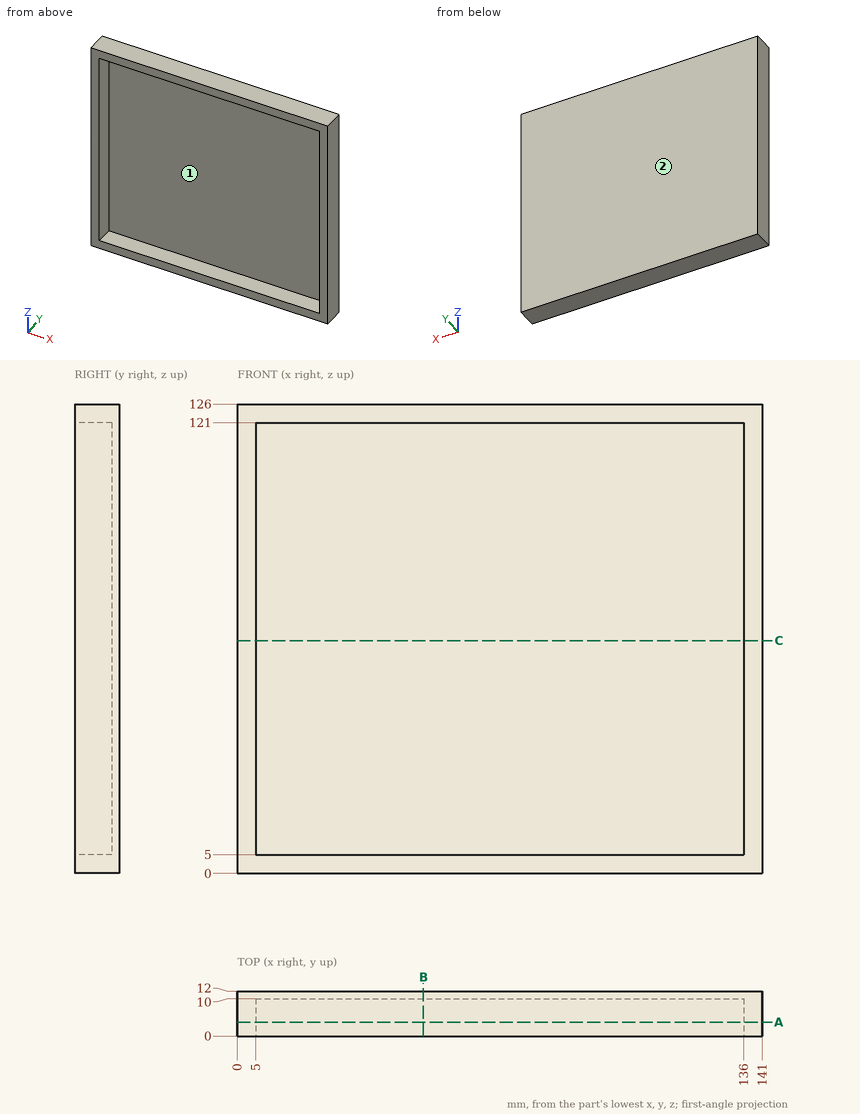
Input: dimensioned drawing with shaded views. Units: mm. Origin: part minimum x, y, z. Give positions to 0.01 mm unless a question says otherwise; leave off trailing zeros. Loops run counter-clockwise (first coordinate to the right, second up) from the corner with the lowest first, then second, coordinate; pieces in that order, holes last. Notation, with made-up numbers: M 18,46.5 L 56,46.5 A17 ccw 56,72.5 Z; hole C 74.25,-35.75 d10. An arc over 180 degrees is marked long. Put each result on its own line as item: value. Start each with the question number.
1) Cut plane A-A (y = 3.75). Output: boundary loops of the cut face in (x, z), then the cut area to 3 significant figures.
2) Ray query, line 1 along X through (y, z) = (6, 44); line 2 along Z through (x, y) = (105, 2.5); line 3 along Y through (x, z) = (110, 100). Return the intervals inside material, ascending.
3) Contact query for flat-ended pins moving along their axis: pin 1 (1.5 mm diameter, centred on y = 4, z = 55.5, fed in from -X); pin 2 (5 mm diameter, centred on x = 62.5, z = 95.5, fed in from -Y). Output: stop coordinate, or through.
4) Cut plane B-B (x = 50). Output: boundary loops of the cut face in (y, z).
5) Cut plane C-C (z = 62.5). Output: boundary loops of the cut face in (x, y), then the cut area to 3 significant figures.
6) Pull-direction query (Z, two-part tool) for the marked faces 1 and 2; classes: pulls with the +Z half, pulls with the -Z half, needs draft (parallel to the pull), parting line crosses it, or undercut.
Verdict:
1. outline: M 0,0 L 141,0 L 141,126 L 0,126 Z; hole M 5,5 L 136,5 L 136,121 L 5,121 Z
1. area: 2,570 mm2
2. line 1: 0 to 5, 136 to 141
2. line 2: 0 to 5, 121 to 126
2. line 3: 10 to 12
3. pin 1: x = 0
3. pin 2: y = 10
4. outline: M 0,0 L 12,0 L 12,126 L 0,126 L 0,121 L 10,121 L 10,5 L 0,5 Z
5. outline: M 0,0 L 5,0 L 5,10 L 136,10 L 136,0 L 141,0 L 141,12 L 0,12 Z
5. area: 382 mm2
6. face 1: undercut
6. face 2: needs draft
